The model under review builds one solid part; all positions refer to its coordinate system, in mm. A direction names the side the tool comes from. Coordinates: 2 decimals unless noted, no trailing zeros. Write each loop counter-clockwise with the first axis right and the second up, starting at its lowest first coordinate (ties: lowest second). Pieces come first, ordered by that corner, then holes. Notation, with made-up numbers: (46.25, 78) - (102.25, 78) arc R15 ccw to (102.25, 88) - close; hole circle Ø4 at (-0.75, 33.5). An arc over 180 degrees is marked (long way). Return JSON: item names as keys, results as strings. Group by question number.
(1) To check wall thickness, follow L1, parallel to X at y = 14, z = 5; L2, parallel to Y at x = 1, z = 2; L3, parallel to Y at x = 20, z = 1. State the ranges of each line that lie inside material, in increasing order. Write a range as from..to.
(2) Draft analysis for pull direction Y (two halves, no side actions). For faces 4 (the face through (24, -1.27, 3)), 5 (the face through (-9.5, -9.4, 0)), 6 (the face through (0, 43.18, 3)), state which applies: released by +Y, released by -Y, zero draft, split by the parting line, or undercut.
(3) We need section B-B on y = 38.5. State the section outline as (x, z) points, then the cut area to 3 significant figures.
(4) For pin 1 Ø2 at (x, z) = (23, 2) entering from -Y; pin 2 Ø10 at (x, y) = (-22, 18) entering from -Z; pin 3 Ø3 at (x, z) = (-21, 2.5) entering from +Y, all flat-tipped, find the tip position at first contact; note any pin that passes through.
(5) Tool access review of faces 1 (the face through (25, 29.21, 3)), 2 (the face through (-35.247, -7.709, 3.131)), 3 (the face through (37.819, 7.085, 3.131)): name each direction out of +Z, -Z, +X, -X, +Y, -Y from which nothing blocks a thin tool from reaching the whole face with its end or side.
(6) We need section D-D on y = 8.5. State the section outline as (x, z) points, then the cut area to 3 significant figures.
(7) We need section A-A on x = -0.5. State the section outline as (y, z) points, then the cut area to 3 significant figures.
(8) We need section C-C on x = -12. State the section outline as (y, z) points, then the cut area to 3 significant figures.
```python
from build123d import *

# Parameters (mm, degrees)
F1_DEPTH = 6.35


with BuildPart() as f1:
    # F0 (on Top) → F1 (new body)
    with BuildSketch(Plane.XY):
        Polygon((31.529098, 26.67), (16.864401, 26.67), (9.532053, 13.97), (16.864401, 1.27), (31.342068, 1.27), (31.529098, 1.27), (38.861447, 13.97), align=None)
        Polygon((41.794386, 13.97), (32.995568, 29.21), (17.544992, 29.21), (16.524106, 29.799409), (8.798818, 43.18), (-8.798818, 43.18), (-16.524106, 29.799409), (-17.544992, 29.21), (-32.995568, 29.21), (-41.794386, 13.97), (-34.069098, 0.589409), (-34.069098, -0.589409), (-41.794386, -13.97), (-32.995568, -29.21), (-17.544992, -29.21), (-16.524106, -29.799409), (-8.798818, -43.18), (8.798818, -43.18), (16.524106, -29.799409), (17.544992, -29.21), (32.995568, -29.21), (41.794386, -13.97), (34.01954, -0.503571), (33.953768, 0.389652), align=None)
        Polygon((7.332348, -15.24), (14.664697, -27.94), (7.332348, -40.64), (-7.332348, -40.64), (-14.664697, -27.94), (-7.332348, -15.24), align=None, mode=Mode.SUBTRACT)
        Polygon((-9.532053, -13.97), (-16.864401, -26.67), (-31.529098, -26.67), (-38.861447, -13.97), (-31.529098, -1.27), (-16.864401, -1.27), align=None, mode=Mode.SUBTRACT)
        Polygon((16.864401, -1.27), (31.529098, -1.27), (38.861447, -13.97), (31.529098, -26.67), (16.864401, -26.67), (9.532053, -13.97), align=None, mode=Mode.SUBTRACT)
        Polygon((-16.864401, 1.27), (-31.529098, 1.27), (-38.861447, 13.97), (-31.529098, 26.67), (-16.864401, 26.67), (-9.532053, 13.97), align=None, mode=Mode.SUBTRACT)
        Polygon((14.664697, 0), (7.332348, -12.7), (-7.332348, -12.7), (-14.664697, 0), (-7.332348, 12.7), (7.332348, 12.7), align=None, mode=Mode.SUBTRACT)
        Polygon((9.532053, 13.97), (16.864401, 26.67), (31.529098, 26.67), (38.861447, 13.97), (31.529098, 1.27), (31.342068, 1.27), (16.864401, 1.27), align=None, mode=Mode.SUBTRACT)
        Polygon((14.664697, 27.94), (7.332348, 15.24), (-7.332348, 15.24), (-14.664697, 27.94), (-7.332348, 40.64), (7.332348, 40.64), align=None, mode=Mode.SUBTRACT)
    extrude(amount=F1_DEPTH)


solid = f1.part
```
Ans:
{
 "1": {"L1": "-41.78..-38.84, -9.55..9.55, 38.84..41.78", "L2": "-43.18..-40.64, -15.24..-12.7, 12.7..15.24, 40.64..43.18", "L3": "-29.21..-26.67, -1.27..1.27, 26.67..29.21"},
 "2": {"face 4": "undercut", "face 5": "zero draft", "face 6": "released by +Y"},
 "3": {"outline": "(-11.5, 0) - (-8.57, 0) - (-8.57, 6.35) - (-11.5, 6.35) - close; (8.57, 0) - (11.5, 0) - (11.5, 6.35) - (8.57, 6.35) - close", "area": "37.2 mm²"},
 "4": {"pin 1": "y = -29.21", "pin 2": "through", "pin 3": "y = 29.21"},
 "5": {"face 1": "+Z, -Z, +X, +Y", "face 2": "+Z, -Z", "face 3": "+Z, -Z, +X"},
 "6": {"outline": "(-38.64, 0) - (-35.7, 0) - (-35.7, 6.35) - (-38.64, 6.35) - close; (-12.69, 0) - (-9.76, 0) - (-9.76, 6.35) - (-12.69, 6.35) - close; (9.76, 0) - (12.69, 0) - (12.69, 6.35) - (9.76, 6.35) - close; (35.7, 0) - (38.64, 0) - (38.64, 6.35) - (35.7, 6.35) - close", "area": "74.5 mm²"},
 "7": {"outline": "(-43.18, 0) - (-40.64, 0) - (-40.64, 6.35) - (-43.18, 6.35) - close; (-15.24, 0) - (-12.7, 0) - (-12.7, 6.35) - (-15.24, 6.35) - close; (12.7, 0) - (15.24, 0) - (15.24, 6.35) - (12.7, 6.35) - close; (40.64, 0) - (43.18, 0) - (43.18, 6.35) - (40.64, 6.35) - close", "area": "64.5 mm²"},
 "8": {"outline": "(-37.64, 0) - (-32.56, 0) - (-32.56, 6.35) - (-37.64, 6.35) - close; (-23.32, 0) - (-18.24, 0) - (-18.24, 6.35) - (-23.32, 6.35) - close; (-9.7, 0) - (-4.62, 0) - (-4.62, 6.35) - (-9.7, 6.35) - close; (4.62, 0) - (9.7, 0) - (9.7, 6.35) - (4.62, 6.35) - close; (18.24, 0) - (23.32, 0) - (23.32, 6.35) - (18.24, 6.35) - close; (32.56, 0) - (37.64, 0) - (37.64, 6.35) - (32.56, 6.35) - close", "area": "194 mm²"}
}
